from build123d import *

# Parameters (mm, degrees)
EXTRUDE_THIN1_DEPTH = 101.6
SKETCH3_R           = 9.525
EXTRUDE1_DEPTH      = 101.6
SKETCH2_R           = 12.7
SKETCH2_R_2         = 9.525
EXTRUDE2_DEPTH      = 45.085
EXTRUDE3_DEPTH      = 101.6


with BuildPart() as part:
    # Sketch1 → Extrude-Thin1 (new body)
    with BuildSketch(Plane(origin=(0, 0, 0), x_dir=(1, 0, 0), z_dir=(0, 1, 0))):
        with BuildLine():
            Line((0, 0), (0, 61.221397696))
            ThreePointArc((0, 61.221397696), (5.35372705, 69.204377703), (14.771330869, 67.281072892))
            ThreePointArc((14.771330869, 67.281072892), (23.8125, 63.5), (32.853669131, 67.281072892))
            ThreePointArc((32.853669131, 67.281072892), (42.27127295, 69.204377703), (47.625, 61.221397696))
            Line((47.625, 61.221397696), (47.625, 0))
            Line((47.625, 0), (45.085, 0))
            Line((45.085, 0), (45.085, 61.221397696))
            ThreePointArc((45.085, 61.221397696), (41.307248552, 66.854429414), (34.661902957, 65.497287471))
            ThreePointArc((34.661902957, 65.497287471), (23.8125, 60.96), (12.963097043, 65.497287471))
            ThreePointArc((12.963097043, 65.497287471), (6.317751448, 66.854429414), (2.54, 61.221397696))
            Line((2.54, 61.221397696), (2.54, 0))
            Line((2.54, 0), (0, 0))
        make_face()
    extrude(amount=-EXTRUDE_THIN1_DEPTH)

    # Sketch3 → Extrude1 (cut)
    with BuildSketch(Plane.ZY):
        with Locations((-41.275, -41.91)):
            Circle(SKETCH3_R)
    extrude(amount=-EXTRUDE1_DEPTH, mode=Mode.SUBTRACT)

    # Sketch2 → Extrude2 (add)
    with BuildSketch(Plane.ZY):
        with Locations((-41.275, -41.91)):
            Circle(SKETCH2_R)
        with Locations((-41.275, -41.91)):
            Circle(SKETCH2_R_2, mode=Mode.SUBTRACT)
    extrude(amount=-EXTRUDE2_DEPTH)

    # Sketch4 → Extrude3 (cut)
    with BuildSketch(Plane.ZY):
        with BuildLine():
            Line((-25.053018977, -15.684280765), (0, -76.2))
            Line((0, -76.2), (0, 0))
            Line((0, 0), (-48.521397696, 0))
            ThreePointArc((-48.521397696, 0), (-34.407915996, -4.282006859), (-25.053018977, -15.684280765))
        make_face()
        with BuildLine():
            ThreePointArc((0, -76.2), (-7.439487758, -94.160512242), (-25.4, -101.6))
            Line((-25.4, -101.6), (0, -101.6))
            Line((0, -101.6), (0, -76.2))
        make_face()
    extrude(amount=-EXTRUDE3_DEPTH, mode=Mode.SUBTRACT)


solid = part.part
For this review, take the finished solid that the model builds, in its own axes (mm). A direction names the side the tool comes from. Round coordinates to 2 decimals unless told otherwise and drop trailing zeros. Loops run counter-clockwise (first coordinate to the right, second up) from the corner with the lowest first, then second, coordinate; pieces in that order, holes last. Notation, with made-up numbers: (46, -38.5) - (69, -38.5) arc R13 cw to (69, -25.5) - close; hole circle Ø3 at (6, 63.5). An arc over 180 degrees is marked (long way). Put each result on its own line as item: value. Start each with the question number.
1. For probe 1 along X at (y, z) = (-70, -25.5) (3 decimals); probe 2 along Z at (x, y) = (32, -41); probe 3 along Z at (x, y) = (11.5, -35.5), list the stretches that pass through material, from the lowest coordinate up. Write a range as [from, to].
2. Consider section D-D on z = -35. State the section outline as (x, y) points (3 decimals).
3. Insertion check: P1, Ø4, axis at x = 27, z = -49, coming from the +Y side; P2, Ø1, axis at x = 19, y = -13.5, coming from the +Z side; P3, Ø5, axis at x = 25.5, y = -31.5, coming from the -Z side. Each pin has a flat end and moves straight along its axis. Give the tip position at first contact, or say it passes through.
4. Consider section A-A on y = -41.91. State how many separate pieces and enclosed holes the cut face has, plus the area to 3 significant figures.
5. Consider section B-B on z = -57. State the section outline as (x, y) points (3 decimals).
6. Consider section C-C on y = -61.5. State the section outline as (x, z) points (1 decimal), plus the area to 3 significant figures.
7. Mouldability with a two-part tool opening along X and no side actions: class faces 4 (the flat face through (45.085, -61, -37)), 5 (the cylindrical face through (5.22, -50.09, -69.15)), 6 (the flat face through (0, -61, -37)), 7 (the flat face through (46.34, -45.52, -12.7)) as +X half, -X half, draft (parallel to the pull), parting line (faces both ways), or undercut.
8. For faces 1 (the cylindrical face through (23.7, -50.1, -63.5)), 2 (the cylindrical face through (23.51, -46.77, -29.54)), 3 (the cylindrical face through (41.4, -50.089, -66.815)), list the 3-axis set-ups (+Z, -Z, +X, -X, +Y, -Y) from which the entire face can be reached by the end or side of a thin tool; tool diameter is ignored.
Result sheet:
1. probe 1: [0, 2.54], [45.085, 47.625]
1. probe 2: [-66.49, -63.35], [-53.94, -50.76], [-31.79, -28.61]
1. probe 3: [-69.36, -66.59], [-52.24, -48.32], [-34.23, -30.31]
2. outline: (0, -101.6) - (2.54, -101.6) - (2.54, -52.951) - (45.085, -52.951) - (45.085, -101.6) - (47.625, -101.6) - (47.625, -49.076) - (0, -49.076) - close; (0, -34.744) - (47.625, -34.744) - (47.625, -3.898) - (45.085, -3.898) - (45.085, -30.869) - (2.54, -30.869) - (2.54, -3.898) - (0, -3.898) - close
3. P1: y = -30.57
3. P2: z = -61.58
3. P3: z = -64.21
4. separate pieces: 2
4. enclosed holes: 1
4. area: 557 mm^2
5. outline: (0, -101.6) - (2.54, -101.6) - (2.54, 0) - (0, 0) - close; (45.085, -101.6) - (47.625, -101.6) - (47.625, 0) - (45.085, 0) - close
6. outline: (0, -61.2) arc R8.6 ccw to (14.8, -67.3) arc R12.7 cw to (32.9, -67.3) arc R8.6 ccw to (47.6, -61.2) - (47.6, -6.1) - (45.1, -6.1) - (45.1, -61.2) arc R6.1 cw to (34.7, -65.5) arc R15.2 ccw to (13, -65.5) arc R6.1 cw to (2.5, -61.2) - (2.5, -6.1) - (0, -6.1) - close
6. area: 425 mm^2
7. face 4: undercut
7. face 5: undercut
7. face 6: -X half
7. face 7: draft
8. face 1: -Z, +Y, -Y
8. face 2: none
8. face 3: +Y, -Y
